Here's the drawing with two shaded views (mm, measured from the low corner). I have some questions. A direction names the side the tool comes from. Give positions to 0.01 mm unless a question says otherwise; leave off trailing zeros. Loops run counter-clockwise (first coordinate to the right, second up) from the corner with the lowest first, then second, coordinate; pieces in that order, holes last. Notation, with made-up numbers: (32.25, 40) -> (83.25, 40) arc R35 ccw to (83.25, 77) -> close; hole circle Ø7 at (69.5, 36). An arc over 180 degrees is marked (long way). Write each question's results on one line, items separated by ' | '. Start each with the question number.
Q1. If I drill on line 1 along Y through (x, z) = (7, 75); line 2 along Z through (x, y) = (3.5, 71); line 3 along X through (y, z) = (75.5, 30.5), over which ranges is the centre line in solid material (lowest first)?
Q2. If we section it at A-A, the plane x = 10.75: List the corners of the cut face in (y, z) for me.
Q3. Which directions (+Z, -Z, +X, -X, +Y, -Y) give clear straight access to the entire face, cutting with the end or side of a thin tool? Please do the marked faces 1 and 2.
Q4. Will these pins go through, and if not, where does the flat tip stop? P1, Ø5.5, axis at x = 11, z = 77, coming from the -Y side; P2, Ø4, axis at x = 12, z = 77, coming from the +Y side; P3, Ø4, axis at x = 2, z = 59, coming from the +Y side.
Q5. If we section it at D-D, the plane y = 35: List the corners of the cut face in (x, z) for me.
Q6. If we section it at B-B, the plane y = 61: List the corners of the cut face in (x, z) for me.
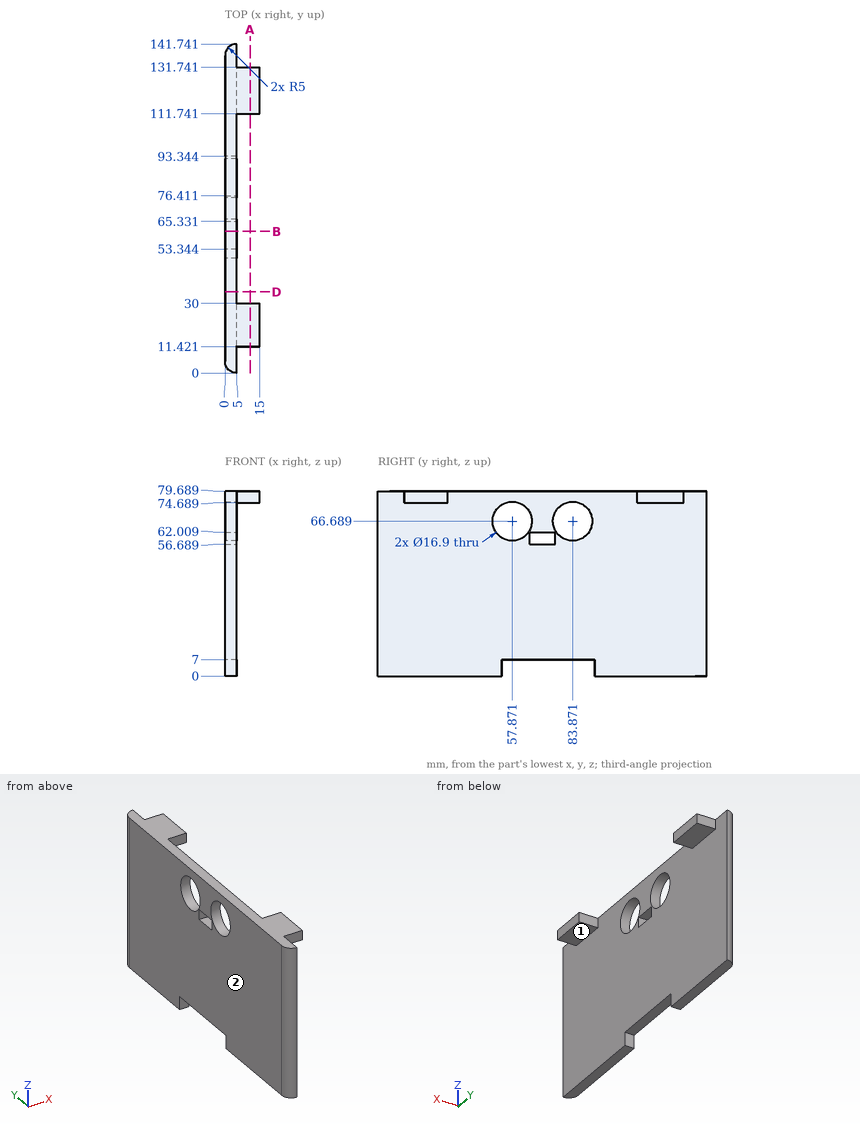
Final values:
1) line 1: y = 11.42 to 30, 111.74 to 131.74 | line 2: z = 7 to 56.69, 62.01 to 79.69 | line 3: x = 0 to 5
2) outline: (11.42, 74.69) -> (30, 74.69) -> (30, 79.69) -> (11.42, 79.69) -> close; (111.74, 74.69) -> (131.74, 74.69) -> (131.74, 79.69) -> (111.74, 79.69) -> close
3) face 1: -Z, +X, +Y, -Y | face 2: +Z, -Z, -X, +Y, -Y
4) P1: stops at y = 11.42 | P2: stops at y = 131.74 | P3: stops at y = 141.64
5) outline: (0, 0) -> (5, 0) -> (5, 79.69) -> (0, 79.69) -> close
6) outline: (0, 7) -> (5, 7) -> (5, 58.84) -> (0, 58.84) -> close; (0, 74.54) -> (5, 74.54) -> (5, 79.69) -> (0, 79.69) -> close
